Part model, mm, in its own coordinate system. A direction names the side the tool comes from. Coordinates: 2 decimals unless noted, no trailing zeros. Loops run counter-clockwise (first coordinate to the right, second up) from the corner with the lowest first, then second, coordinate; pieces in that order, holes last. Notation, with made-up numbers: M -3.5,60 L 6.5,60 A22 ccw 6.5,88 Z; hole C 35,-19 d1. An arc over 180 degrees is marked long. Answer as a JSON object with one key per item and string values. Group by question number.
1. Saw through at B-B on y = -13.5. Write the cut outline in (x, z), then the cut area to 3 significant figures.
2. Drill centre lines: L1, parallel to Z at x = 45, y = -9; L2, parallel to Y at x = 69, z = 73; L3, parallel to Z at x = -93.5, y = -4.5. Where is each one in solid material? Low to high.
3. Saw through at C-C on z = 73. Write the cut outline in (x, y).
4. Drop flat-ended pins along their axis: pin 1 Ø5 at (x, y) = (-9.5, -13.5) entering from -Z; pin 2 Ø6.5 at (x, z) = (97.94, 53.65) entering from -Y. Give the stop position or say it passes through.
5. Saw through at A-A on x = 81. Write the cut outline in (y, z), then the cut area to 3 significant figures.
6. Mould opens along X. For faces 1 (the face through (100.333, -1.198, 66.661)), 2 (the face through (105.918, -2, 73)), 3 (the face through (-105.918, -2, 50)) say: released by +X, released by -X, zero draft, split by the parting line, or undercut.
7. 3-axis set-ups, long thin cutter, end or side, ignore diameter. For faces 4 (the face through (1, -12, 87.757)), 5 (the face through (-93.546, -1.198, 77.75)): which of +Z, -Z, +X, -X, +Y, -Y reach the whole face in a straight line?
from build123d import *

# Parameters (mm, degrees)
SKETCH1_W                    = 211.836
SKETCH1_H                    = 175.514
BASE_FLANGE1_DEPTH           = 2.3622
EDGE_FLANGE4_STRIP_W         = 14.1688
EDGE_FLANGE4_STRIP_H         = 2.3622
EDGE_FLANGE4_STRIP_CUT_DEPTH = 211.836
EDGE_FLANGE4_DEPTH           = 211.836
CUT_EXTRUDE1_DEPTH           = 141.066325723
SKETCH38_R                   = 2.413
CUT_EXTRUDE3_DEPTH           = 141.066325723
SKETCH40_R                   = 2.413
CUT_EXTRUDE4_DEPTH           = 141.066325723


# Sheet-metal steps are written as plain solids
with BuildPart() as part:
    # Sketch1 → Base-Flange1 (new body)
    with BuildSketch(Plane(origin=(0, 0, 0), x_dir=(1, 0, 0), z_dir=(0, 1, 0))):
        Rectangle(SKETCH1_W, SKETCH1_H)
    extrude(amount=-BASE_FLANGE1_DEPTH)

    # Edge-Flange4 strip (across the edge) → Edge-Flange4 strip cut (cut)
    with BuildSketch(Plane(origin=(105.918, -2.3622, 87.757), x_dir=(0, 0, -1), z_dir=(-1, 0, 0))):
        with Locations((-4.7244, -1.1811)):
            Rectangle(EDGE_FLANGE4_STRIP_W, EDGE_FLANGE4_STRIP_H)
    extrude(amount=EDGE_FLANGE4_STRIP_CUT_DEPTH, mode=Mode.SUBTRACT)

    # Edge-Flange4 section (across the edge) → Edge-Flange4 (add)
    with BuildSketch(Plane(origin=(105.918, -2.3622, 87.757), x_dir=(0, 0, -1), z_dir=(-1, 0, 0))):
        with BuildLine():
            Line((-2.3622, 2.36), (-2.3622, 16.6878))
            Line((-2.3622, 16.6878), (0, 16.6878))
            Line((0, 16.6878), (0, 2.36))
            ThreePointArc((0, 2.36), (0.691227996, 0.691227996), (2.36, 0))
            Line((2.36, 0), (2.36, -2.3622))
            ThreePointArc((2.36, -2.3622), (-0.979099642, -0.979099642), (-2.3622, 2.36))
        make_face()
    extrude(amount=EDGE_FLANGE4_DEPTH)

    # Sketch36 → Cut-Extrude1 (cut, through all)
    with BuildSketch(Plane.XZ.offset(2.3622)):
        Polygon((28.702, -11.4808), (-105.918, -11.4808), (-105.918, -87.757), (105.918, -87.757), (105.918, 47.2567), align=None)
    extrude(amount=-CUT_EXTRUDE1_DEPTH, mode=Mode.SUBTRACT)

    # Sketch38 → Cut-Extrude3 (cut, through all)
    with BuildSketch(Plane.XZ.offset(2.3622)):
        with Locations(Location((97.9402, 79.047, 0), (0, 0, 270))):
            Circle(SKETCH38_R)
        with Locations(Location((97.9402, 66.347, 0), (0, 0, 270))):
            Circle(SKETCH38_R)
        with Locations(Location((97.9402, 53.647, 0), (0, 0, 270))):
            Circle(SKETCH38_R)
    extrude(amount=-CUT_EXTRUDE3_DEPTH, mode=Mode.SUBTRACT)

    # Sketch40 → Cut-Extrude4 (cut, through all)
    with BuildSketch(Plane.XZ.offset(2.3622)):
        with Locations(Location((-95.5802, 79.047, 0), (0, 0, 270))):
            Circle(SKETCH40_R)
        with Locations(Location((-95.5802, 64.7595, 0), (0, 0, 270))):
            Circle(SKETCH40_R)
        with Locations(Location((-95.5802, 50.472, 0), (0, 0, 270))):
            Circle(SKETCH40_R)
        with Locations(Location((-95.5802, 36.1845, 0), (0, 0, 270))):
            Circle(SKETCH40_R)
        with Locations(Location((-95.5802, 21.897, 0), (0, 0, 270))):
            Circle(SKETCH40_R)
        with Locations(Location((-95.5802, 7.6095, 0), (0, 0, 270))):
            Circle(SKETCH40_R)
        with Locations(Location((-95.5802, -6.678, 0), (0, 0, 270))):
            Circle(SKETCH40_R)
    extrude(amount=-CUT_EXTRUDE4_DEPTH, mode=Mode.SUBTRACT)


solid = part.part
Outcome:
{
 "1": {"outline": "M -105.92,87.76 L 105.92,87.76 L 105.92,90.12 L -105.92,90.12 Z", "area": "500 mm²"},
 "2": {"L1": "z = 87.76 to 90.12", "L2": "y = -2.36 to 0", "L3": "z = 87.75 to 90.11"},
 "3": {"outline": "M -105.92,-2.36 L 105.92,-2.36 L 105.92,0 L -105.92,0 Z"},
 "4": {"pin 1": "stops at z = 87.76", "pin 2": "stops at y = -2.36"},
 "5": {"outline": "M -19.05,87.76 L -4.72,87.76 A2.36 cw -2.36,85.4 L -2.36,28.3 L 0,28.3 L 0,85.4 A4.72 ccw -4.72,90.12 L -19.05,90.12 Z", "area": "182 mm²"},
 "6": {"face 1": "undercut", "face 2": "released by +X", "face 3": "released by -X"},
 "7": {"face 4": "-Z, +X, -X, -Y", "face 5": "+Y, -Y"}
}
